Source: CAD feature listing. Evaluate the final solid. Frame: model axes, mm. Give positions to 0.01 mm unless a question says otherwise; leave off trailing zeros. Write each loop counter-clockwise with the first axis right and the second up, starting at its lowest first coordinate (ties: lowest second). Pieces come first, ordered by that corner, then holes. Notation, with made-up numbers: (13, 88) -> (69, 88) arc R27 ccw to (69, 124) -> close; hole circle Ø8 at (62, 82.25). An arc over 180 degrees is marked (long way). Use one line per item in the form item = value. Start each with the question number.
(1) Cut plane A-A, the plane z = 4.25. Output: boundary loops of the cut face in (x, y) (1 decimal).
(2) Cut plane B-B, the plane y = -4.75. Output: boundary loops of the cut face in (x, z).
(3) Material intervals for line 1 along X through (y, z) = (-0.5, 0.75); line 2 along X through (y, z) = (-6.25, 4.25); line 3 along Y through (x, z) = (-45.5, 3.5), sorted ascending. Write a range as from..to.
(4) Draft query along Y for faces 1 (the face through (48.627, 5.646, 3.219)), 2 (the face through (33.34, 0.07, 3.22)), 3 (the face through (-48.627, -5.646, 3.219)). Return one class per face: pulls with the +Y half, pulls with the -Y half, needs draft (parallel to the pull), parting line crosses it, or undercut.
(5) Cut plane C-C, the plane y = 6. Output: boundary loops of the cut face in (x, z), and give its area (3 significant figures).
(6) First-contact query: P1, Ø3, axis at x = -34.925, y = 0, coming from the -Z side. Flat tip, straight axial feed; report the tip coordinate or a pass-through.
from build123d import *

# Parameters (mm, degrees)
F0_W     = 101.6
F0_H     = 15.875
F1_DEPTH = 6.35
F2_R     = 7.62
F3_R     = 1.5875
F4_DEPTH = 25.4


with BuildPart() as f1:
    # F0 (on Top) → F1 (new body)
    with BuildSketch(Plane.XY):
        Rectangle(F0_W, F0_H)
    extrude(amount=F1_DEPTH)

    # F2
    f2_edges = [f1.edges().sort_by_distance(p)[0] for p in [
        (-50.8, 7.9375, 3.175),
        (-50.8, -7.9375, 3.175),
        (50.8, 7.9375, 3.175),
        (50.8, -7.9375, 3.175),
    ]]
    fillet(f2_edges, radius=F2_R)

    # F3 (on face) → F4 (cut)
    with BuildSketch(Plane.XY.offset(6.35)):
        with Locations((-34.925, 0)):
            Circle(F3_R)
        with Locations((34.925, 0)):
            Circle(F3_R)
    extrude(amount=-F4_DEPTH, mode=Mode.SUBTRACT)


solid = f1.part
Geometry says:
q1.outline = (-50.8, -0.3) arc R7.6 ccw to (-43.2, -7.9) -> (43.2, -7.9) arc R7.6 ccw to (50.8, -0.3) -> (50.8, 0.3) arc R7.6 ccw to (43.2, 7.9) -> (-43.2, 7.9) arc R7.6 ccw to (-50.8, 0.3) -> close; hole circle Ø3.2 at (-34.9, 0); hole circle Ø3.2 at (34.9, 0)
q2.outline = (-49.38, 0) -> (49.38, 0) -> (49.38, 6.35) -> (-49.38, 6.35) -> close
q3.line_1 = -50.8..-36.43, -33.42..33.42, 36.43..50.8
q3.line_2 = -47.96..47.96
q3.line_3 = -7.58..7.58
q4.face_1 = pulls with the +Y half
q4.face_2 = undercut
q4.face_3 = pulls with the -Y half
q5.outline = (-48.26, 0) -> (48.26, 0) -> (48.26, 6.35) -> (-48.26, 6.35) -> close
q5.area = 613 mm^2
q6.P1 = through
